The listing builds one solid part. Answer for the finished solid, in the listing's coordinates (mm). A direction names the side the tool comes from. Coordinates: 2 decimals unless noted, no trailing zeros. Write each loop counter-clockwise with the first axis right and the second up, starting at its lowest first coordinate (ties: lowest second). Pieces come first, ordered by that corner, then holes.
from build123d import *

# Parameters (mm, degrees)
SKETCH_W        = 48
SKETCH_H        = 28
PAD_DEPTH       = 10
SKETCH001_W     = 45.5
SKETCH001_H     = 24.5
POCKET_DEPTH    = 8.5
PAD001_DEPTH    = 6.5
SKETCH003_R     = 0.75
POCKET001_DEPTH = 5
SKETCH004_W     = 9.5
SKETCH004_H     = 5.5
POCKET002_DEPTH = 1.25
SKETCH005_W     = 10.5
SKETCH005_H     = 8
POCKET003_DEPTH = 1.25
FILLET_R        = 1
FILLET001_R     = 1
SKETCH012_R     = 0.75
POCKET007_DEPTH = 1.75
SKETCH013_W     = 3.6
SKETCH013_H     = 2.5
POCKET008_DEPTH = 0.8
SKETCH015_R     = 1.25
POCKET009_DEPTH = 1.501


with BuildPart() as part:
    # Sketch → Pad (new body)
    with BuildSketch(Plane.XY):
        Rectangle(SKETCH_W, SKETCH_H)
    extrude(amount=PAD_DEPTH)

    # Sketch001 (on Face6 of Pad) → Pocket (cut)
    with BuildSketch(Plane.XY.offset(10)):
        Rectangle(SKETCH001_W, SKETCH001_H)
    extrude(amount=-POCKET_DEPTH, mode=Mode.SUBTRACT)

    # Sketch002 (on Face11 of Pocket) → Pad001 (join)
    with BuildSketch(Plane.XY.offset(1.5)):
        with BuildLine():
            Line((-22.75, -6), (-16.5, -6))
            ThreePointArc((-14.75, -7.75), (-15.262563, -6.512563), (-16.5, -6))
            Line((-14.75, -12.25), (-14.75, -7.75))
            Line((-22.75, -12.25), (-14.75, -12.25))
            Line((-22.75, -6), (-22.75, -12.25))
        make_face()
        with BuildLine():
            Line((6, 12.25), (6, 8))
            ThreePointArc((6, 8), (7.75, 6.25), (9.5, 8))
            Line((9.5, 12.25), (9.5, 8))
            Line((6, 12.25), (9.5, 12.25))
        make_face()
    extrude(amount=PAD001_DEPTH)

    # Sketch003 (on Face13 of Pad001) → Pocket001 (cut)
    with BuildSketch(Plane.XY.offset(8)):
        with Locations((-16.5, -7.75)):
            Circle(SKETCH003_R)
        with Locations((7.75, 8)):
            Circle(SKETCH003_R)
    extrude(amount=-POCKET001_DEPTH, mode=Mode.SUBTRACT)

    # Sketch004 (on Face2 of Pocket001) → Pocket002 (cut)
    with BuildSketch(Plane(origin=(-24, 0, 0), x_dir=(0, -1, 0), z_dir=(-1, 0, 0))):
        with Locations((-0.5, 7.25)):
            Rectangle(SKETCH004_W, SKETCH004_H)
    extrude(amount=-POCKET002_DEPTH, mode=Mode.SUBTRACT)

    # Sketch005 (on Face3 of Pocket002) → Pocket003 (cut)
    with BuildSketch(Plane.YZ.offset(24)):
        with Locations((-0.495, 6)):
            Rectangle(SKETCH005_W, SKETCH005_H)
    extrude(amount=-POCKET003_DEPTH, mode=Mode.SUBTRACT)

    # Fillet
    fillet_edges = [part.edges().sort_by_distance(p)[0] for p in [
        (-23.375, 5.25, 4.5),
        (-23.375, -4.25, 4.5),
        (-22.75, -6, 4.75),
        (-14.75, -12.25, 4.75),
        (6, 12.25, 4.75),
        (9.5, 12.25, 4.75),
    ]]
    fillet(fillet_edges, radius=FILLET_R)

    # Fillet001
    fillet001_edges = [part.edges().sort_by_distance(p)[0] for p in [
        (-24, -14, 5),
        (24, -14, 5),
        (0, -14, 0),
        (-24, 0, 0),
        (-24, 14, 5),
        (0, 14, 0),
        (24, 14, 5),
        (24, 0, 0),
    ]]
    fillet(fillet001_edges, radius=FILLET001_R)

    # Sketch012 (on Face15 of Fillet001) → Pocket007 (cut)
    with BuildSketch(Plane.XZ.offset(14)):
        with Locations((-9.75, 7)):
            Circle(SKETCH012_R)
    extrude(amount=-POCKET007_DEPTH, mode=Mode.SUBTRACT)

    # Sketch013 (on Face17 of Pocket007) → Pocket008 (cut)
    with BuildSketch(Plane(origin=(0, -12.25, 0), x_dir=(-1, 0, 0), z_dir=(0, 1, 0))):
        with Locations((9.75, 7)):
            Rectangle(SKETCH013_W, SKETCH013_H)
    extrude(amount=-POCKET008_DEPTH, mode=Mode.SUBTRACT)

    # Sketch015 (on Face31 of Pocket008) → Pocket009 (cut, through all)
    with BuildSketch(Plane.XY.offset(1.5)):
        with Locations((-18, 8)):
            Circle(SKETCH015_R)
        with Locations((2, 8)):
            Circle(SKETCH015_R)
    extrude(amount=-POCKET009_DEPTH, mode=Mode.SUBTRACT)


solid = part.part
Q1. Determine the mould class of faces 4 (the face through (-16.845, 7.521, 0.76)), 5 (the face through (-23.715, 13.699, 5.563)), 6 (the face through (0, 0, 0)) for opening direction X: released by +X, released by -X, zero draft, split by the parting line, or undercut.
Answers below:
face 4: undercut
face 5: released by -X
face 6: zero draft
Q2. The part is cut by section C-C, the plane z = 8.75. Write down the section's boundary in (x, y) (3 decimals).
Answers below:
outline: (-24, -13) arc R1 ccw to (-23, -14) - (23, -14) arc R1 ccw to (24, -13) - (24, -5.745) - (22.75, -5.745) - (22.75, -12.25) - (-22.75, -12.25) - (-22.75, -4.25) - (-24, -4.25) - close; (-24, 5.25) - (-22.75, 5.25) - (-22.75, 12.25) - (22.75, 12.25) - (22.75, 4.755) - (24, 4.755) - (24, 13) arc R1 ccw to (23, 14) - (-23, 14) arc R1 ccw to (-24, 13) - close
Q3. The part is cut by section B-B, the plane y = 10. Write down the section's boundary in (x, z).
Answers below:
outline: (-24, 1) arc R1 ccw to (-23, 0) - (23, 0) arc R1 ccw to (24, 1) - (24, 10) - (22.75, 10) - (22.75, 1.5) - (9.5, 1.5) - (9.5, 8) - (6, 8) - (6, 1.5) - (-22.75, 1.5) - (-22.75, 10) - (-24, 10) - close
Q4. Which of the six approach directions +Z, -Z, +X, -X, +Y, -Y give full straight-line access (tool end or side, diameter ignored) to faces 1 (the face through (-23, 1, 4.5)), 2 (the face through (0, 14, 5)), 3 (the face through (0, 12.25, 6))?
Answers below:
face 1: +Z, +X, -X
face 2: +Z, -Z, +X, -X, +Y
face 3: +Z
Q5. The part is cut by section D-D, the plane x = -9.75. Write down the section's boundary in (y, z).
Answers below:
outline: (-14, 1) arc R1 ccw to (-13, 0) - (13, 0) arc R1 ccw to (14, 1) - (14, 10) - (12.25, 10) - (12.25, 1.5) - (-12.25, 1.5) - (-12.25, 5.75) - (-13.05, 5.75) - (-13.05, 6.25) - (-14, 6.25) - close; (-14, 7.75) - (-13.05, 7.75) - (-13.05, 8.25) - (-12.25, 8.25) - (-12.25, 10) - (-14, 10) - close
Q6. The part is cut by section A-A, the plane x = 2. Write down the section's boundary in (y, z).
Answers below:
outline: (-14, 1) arc R1 ccw to (-13, 0) - (6.75, 0) - (6.75, 1.5) - (-12.25, 1.5) - (-12.25, 10) - (-14, 10) - close; (9.25, 0) - (13, 0) arc R1 ccw to (14, 1) - (14, 10) - (12.25, 10) - (12.25, 1.5) - (9.25, 1.5) - close
Q7. Given pin 1 (0.9 mm diameter, centred on x = -16.5, y = -7.75, fed in from +Z); pin 2 (4 mm diameter, centred on y = 2.5, z = 8.5, fed in from -X); pin 3 (1.6 mm diameter, centred on x = 6.5, y = 8, fed in from +Z); pin 4 (1 mm diameter, centred on x = 23.5, y = -2, fed in from +Z), each flat-ended and moving along its own axis, determine where each tip first touches the part or whether it passes through.
Answers below:
pin 1: stops at z = 3
pin 2: passes through
pin 3: stops at z = 8
pin 4: stops at z = 2
Q8. Find the intervals of material crossed by probe 1 along Y at (x, z) = (-16.5, 6.1); probe 2 along Y at (x, z) = (7.75, 4.65); probe 3 along Y at (x, z) = (-18, 1), in increasing order.
Answers below:
probe 1: y = -14 to -8.5, -7 to -6, 12.25 to 14
probe 2: y = -14 to -12.25, 6.25 to 7.25, 8.75 to 14
probe 3: y = -14 to 6.75, 9.25 to 14
